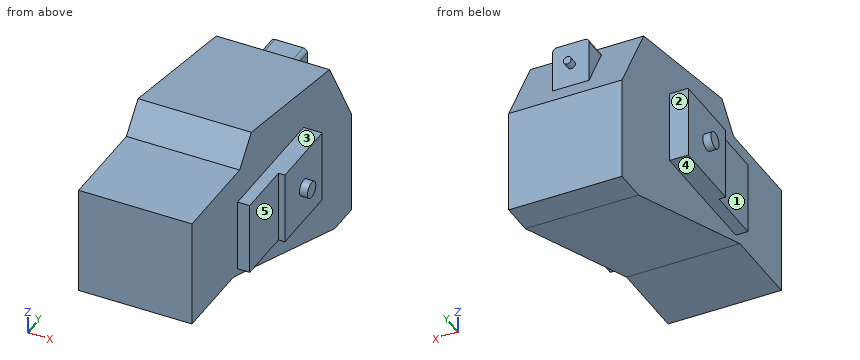
from build123d import *

# Parameters (mm, degrees)
BOSS_EXTRUDE1_DEPTH = 140
BOSS_EXTRUDE2_REACH = 428.071
SKETCH2_W           = 45
SKETCH2_H           = 60
FILLET3_R           = 5
SKETCH3_R           = 4.9
BOSS_EXTRUDE3_DEPTH = 10
SKETCH5_W           = 90
SKETCH5_H           = 159.320081404
BOSS_EXTRUDE4_DEPTH = 15
SKETCH6_W           = 90
SKETCH6_H           = 90
BOSS_EXTRUDE5_DEPTH = 8
SKETCH7_R           = 10
BOSS_EXTRUDE6_DEPTH = 10


with BuildPart() as part:
    # Sketch1 → Boss-Extrude1 (new body)
    with BuildSketch(Plane(origin=(0, 0, 0), x_dir=(0, 0, -1), z_dir=(1, 0, 0))):
        Polygon((-28.65072374, 264.999954135), (101.34927626, 264.999954135), (101.34927626, 224.999954135), (12.424038995, -19.320127269), (12.424038995, -119.320127269), (-122.575961005, -119.320127269), (-122.575961005, -4.320127269), (-155.703127425, 23.841926011), (-121.056779311, 212.517254187), align=None)
    extrude(amount=-BOSS_EXTRUDE1_DEPTH)

    # Boss-Extrude2: up to this face of the body (flat: up to its plane)
    boss_extrude2_end = Plane(part.part.faces().sort_by_distance((-70, 238.758604161, 74.853751525))[0])
    # Sketch2 → Boss-Extrude2 (add, up to the picked face)
    with BuildSketch(Plane(origin=(0, 251.749954135, 0), x_dir=(1, 0, 0), z_dir=(0, 1, 0)), mode=Mode.PRIVATE) as boss_extrude2_sk1:
        with Locations((-70, -78.65072374)):
            Rectangle(SKETCH2_W, SKETCH2_H)
    boss_extrude2_tool1 = split(extrude(boss_extrude2_sk1.sketch, amount=-BOSS_EXTRUDE2_REACH, mode=Mode.PRIVATE), bisect_by=boss_extrude2_end, keep=Keep.BOTH, mode=Mode.PRIVATE)
    add(boss_extrude2_tool1.solids().sort_by(Axis((-70, 251.749954, 78.650724), (0, -1, 0)))[0])

    # Fillet3
    fillet3_edges = [part.edges().sort_by_distance(p)[0] for p in [
        (-47.5, 235.656659485, 108.65072374),
        (-92.5, 235.656659485, 108.65072374),
    ]]
    fillet(fillet3_edges, radius=FILLET3_R)

    # Sketch3 → Boss-Extrude3 (add)
    with BuildSketch(Plane(origin=(0, 251.749954135, 0), x_dir=(1, 0, 0), z_dir=(0, 1, 0))):
        with Locations(Location((-70.732233047, -79.583098626, 0), (0, 0, 270))):
            Circle(SKETCH3_R)
    extrude(amount=BOSS_EXTRUDE3_DEPTH)

    # Sketch5 → Boss-Extrude4 (add)
    with BuildSketch(Plane(origin=(0, 0, 0), x_dir=(0, 0, -1), z_dir=(1, 0, 0))):
        with Locations((-37.575961005, 70.339913433)):
            Rectangle(SKETCH5_W, SKETCH5_H)
    boss_extrude4 = extrude(amount=BOSS_EXTRUDE4_DEPTH)

    # Sketch6 → Boss-Extrude5 (add)
    with BuildSketch(Plane(origin=(15, 0, 0), x_dir=(0, 0, -1), z_dir=(1, 0, 0))):
        with Locations((-37.575961005, 104.999954135)):
            Rectangle(SKETCH6_W, SKETCH6_H)
    boss_extrude5 = extrude(amount=BOSS_EXTRUDE5_DEPTH)

    # Sketch7 → Boss-Extrude6 (add)
    with BuildSketch(Plane(origin=(23, 0, 0), x_dir=(0, 0, -1), z_dir=(1, 0, 0))):
        with Locations((-37.575961005, 104.999954135)):
            Circle(SKETCH7_R)
    boss_extrude6 = extrude(amount=BOSS_EXTRUDE6_DEPTH)

    # Mirror1: Boss-Extrude4, Boss-Extrude5, Boss-Extrude6 across plane
    add(boss_extrude4.mirror(Plane(origin=(-70, 0, 0), x_dir=(0, 0, 1), z_dir=(1, 0, 0))))
    add(boss_extrude5.mirror(Plane(origin=(-70, 0, 0), x_dir=(0, 0, 1), z_dir=(1, 0, 0))))
    add(boss_extrude6.mirror(Plane(origin=(-70, 0, 0), x_dir=(0, 0, 1), z_dir=(1, 0, 0))))


solid = part.part
Geometry check sheet. Reference: the model listing, model coordinates, mm. Face numbers are marked on the shaded views. A direction names the side the tool comes from. Round coordinates to 2 decimals unless told otherwise and drop trailing zeros. Loops run counter-clockwise (first coordinate to the right, second up) from the corner with the lowest first, then second, coordinate; pieces in that order, holes last.
Item 1: Cross-section at D-D on z = 92. Record the boundary of the cut face in (x, y).
Item 2: Cross-section at C-C on z = 65.5. Record the boundary of the cut face in (x, y).
Item 3: Thickness scan on line 1 (X direction, y = 63, z = 33); line 2 (Z direction, x = -81, y = -48.5); line 3 (X direction, y = 166.5, z = -47.5). Record the ranges inside material, lowest first.
Item 4: Access from +Z, -Z, +X, -X, +Y, -Y to the whole of each face (thin tool, end or side, straight path). Record for the marked faces 1, 2, 3, 4 and 5.
Item 5: Cross-section at B-B on y = 230.5. Record the boundary of the cut face in (x, z).
Item 6: Cross-section at A-A on x = -112. Record the boundary of the cut face in (y, z).
Item 7: Gauge pin test, flat ends, axial feed: pin 1 (3 mm diameter, centred on y = -59.5, z = 26.5, fed in from -X); pin 2 (4 mm diameter, centred on y = 8, z = 59.5, fed in from -X); pin 3 (4 mm diameter, centred on x = -148.5, y = 24, fed in from +Z). Record the tip position at first contact, or that the pin passes through.
Answer sheet:
1. outline: (-140, -119.32) - (0, -119.32) - (0, 229.02) - (-47.5, 229.02) - (-47.5, 251.75) - (-92.5, 251.75) - (-92.5, 229.02) - (-140, 229.02) - close
2. outline: (-163, 60) - (-155, 60) - (-155, -9.32) - (-140, -9.32) - (-140, -119.32) - (0, -119.32) - (0, -9.32) - (15, -9.32) - (15, 60) - (23, 60) - (23, 150) - (0, 150) - (0, 244.07) - (-47.5, 244.07) - (-47.5, 251.75) - (-92.5, 251.75) - (-92.5, 244.07) - (-140, 244.07) - (-140, 150) - (-163, 150) - close
3. line 1: x = -163 to 23
3. line 2: z = -12.42 to 122.58
3. line 3: x = -140 to 0
4. face 1: +Z, -Z, -X, -Y
4. face 2: +Z, -Z, -X, +Y
4. face 3: +Z, +X, +Y, -Y
4. face 4: -Z, -X, +Y, -Y
4. face 5: +Z, -Z, +X, -Y
5. outline: (-140, -101.35) - (0, -101.35) - (0, 89.39) - (-47.5, 89.39) - (-47.5, 103.65) arc R5 ccw to (-52.5, 108.65) - (-87.5, 108.65) arc R5 ccw to (-92.5, 103.65) - (-92.5, 89.39) - (-140, 89.39) - close
6. outline: (-119.32, -12.42) - (-19.32, -12.42) - (225, -101.35) - (265, -101.35) - (265, 28.65) - (212.52, 121.06) - (23.84, 155.7) - (-4.32, 122.58) - (-119.32, 122.58) - close
7. pin 1: stops at x = -140
7. pin 2: stops at x = -155
7. pin 3: stops at z = 82.58
